Verification items for the finished model (mm, model axes). Face numbers are marked on the shaded views. A direction names the side the tool comes from. Give positions to 0.01 mm unless a question says otherwise; leave off trailing zeros. Write each loop counter-clockwise with the first axis right and the second up, starting at its lowest first coordinate (ties: lowest second). Pieces come first, ordered by that corner, then holes. Notation, with made-up numbers: M 60,-24 L 114,-24 A25 cw 114,8 Z; hole C 14,45 d1. An arc over 180 degrees is marked long. Answer as a JSON object with one key per item and string values.
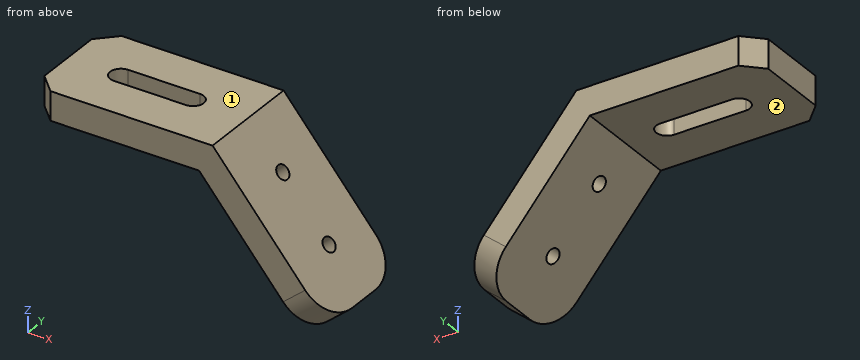
```python
from build123d import *

# Parameters (mm, degrees)
F1_DEPTH = 15
F3_DEPTH = 43.4455230334
F5_D     = 4
F6_R     = 10
F7_SIZE  = 5


with BuildPart() as f1:
    # F0 (on Front) → F1 (new body, symmetric)
    with BuildSketch(Plane.XZ):
        Polygon((0, 8), (0, 0), (46.2695387348, 0), (76.0110249394, -35.4445230334), (82.1393804843, -30.3022221559), (50, 8), align=None)
    extrude(amount=F1_DEPTH, both=True)

    # F2 (on face) → F3 (cut, through all)
    with BuildSketch(Plane.XY.offset(8)):
        with BuildLine():
            ThreePointArc((14.6969384567, 3), (11.6969384567, 0), (14.6969384567, -3))
            Line((14.6969384567, -3), (34.6969384567, -3))
            ThreePointArc((34.6969384567, -3), (37.6969384567, 0), (34.6969384567, 3))
            Line((34.6969384567, 3), (14.6969384567, 3))
        make_face()
    extrude(amount=-F3_DEPTH, mode=Mode.SUBTRACT)

    # F5 (through all)
    with Locations(Plane(origin=(33.2804354537, 0, 27.9256011146), x_dir=(0, 1, 0), z_dir=(0.7660444431, 0, 0.6427876097))):
        with Locations((0, -41.0110249394), (0, -61.0110249394)):
            Hole(F5_D / 2)

    # F6
    f6_edges = [f1.edges().sort_by_distance(p)[0] for p in [
        (79.075203, -15, -32.873373),
        (79.075203, 15, -32.873373),
    ]]
    fillet(f6_edges, radius=F6_R)

    # F7
    f7_edges = [f1.edges().sort_by_distance(p)[0] for p in [
        (0, 15, 4),
        (0, -15, 4),
    ]]
    chamfer(f7_edges, length=F7_SIZE)


solid = f1.part
```
1) Thickness scan on L1, parallel to Z at x = 20, y = 13; L2, parallel to Y at x = 59, z = -5.5; L3, parallel to X at y = 1, z = 6. Record the ranges inside material, lowest first.
Completed:
{"L1": "z = 0 to 8", "L2": "y = -15 to -1.65, 1.65 to 15", "L3": "x = 0 to 11.87, 37.53 to 51.68"}
2) Go/stop test with flat-tipped pins: pin 1 (4 mm diameter, centred on x = 12, y = 9.5, fed in from -Z); pin 2 (2 mm diameter, centred on y = -5.5, z = -4.5, fed in from -X); pin 3 (12 mm diameter, centred on x = 50.5, z = -22.5, fed in from -Y); pin 4 (6 mm diameter, centred on y = 6.5, z = 2, fed in from +X). Record where each tip stops, or that it passes through.
Completed:
{"pin 1": "stops at z = 0", "pin 2": "stops at x = 49.21", "pin 3": "passes through", "pin 4": "stops at x = 57.55"}
3) Section check B-B on y = 0.5. Record the boundary of the cut face in (x, z) (3 decimals), and give its area (3 significant figures).
Completed:
{"outline": "M 0,0 L 11.739,0 L 11.739,8 L 0,8 Z; M 37.655,0 L 46.27,0 L 52.269,-7.15 L 58.397,-2.007 L 50,8 L 37.655,8 Z; M 54.758,-10.116 L 65.124,-22.47 L 71.253,-17.328 L 60.887,-4.974 Z; M 67.614,-25.437 L 76.011,-35.445 L 82.139,-30.302 L 73.742,-20.295 Z", "area": "501 mm2"}
4) Access from +Z, -Z, +X, -X, +Y, -Y to the whole of each face (thin tool, end or side, straight path). Record for the marked faces 1 and 2.
Completed:
{"face 1": "+Z, +X, -X, +Y, -Y", "face 2": "-Z, -X, +Y, -Y"}
5) Section check A-A on x = 22.5. Record the boundary of the cut face in (y, z).
Completed:
{"outline": "M -15,0 L -3,0 L -3,8 L -15,8 Z; M 3,0 L 15,0 L 15,8 L 3,8 Z"}
6) Section check D-D on z = -16. Record the boundary of the cut face in (x, y).
Completed:
{"outline": "M 59.7,-15 L 70.14,-15 L 70.14,15 L 59.7,15 Z"}
7) Section check C-C on x = 10.5. Record the boundary of the cut face in (y, z), and give its area (3 significant figures).
Completed:
{"outline": "M -15,0 L 15,0 L 15,8 L -15,8 Z", "area": "240 mm2"}
